Design review of the part shown in the three views and the two pictorial views. Dimensions are in mm from the part's minimum x, y and z. A direction names the side the tool comes from. Give positions to 0.01 mm unless a question says otherwise; leave off trailing zeros. Order: outer loops, then holes, each group sorted by start corner. A loop starts at its lowest first (then second) coordinate and runs counter-clockwise, first axis right, second up.
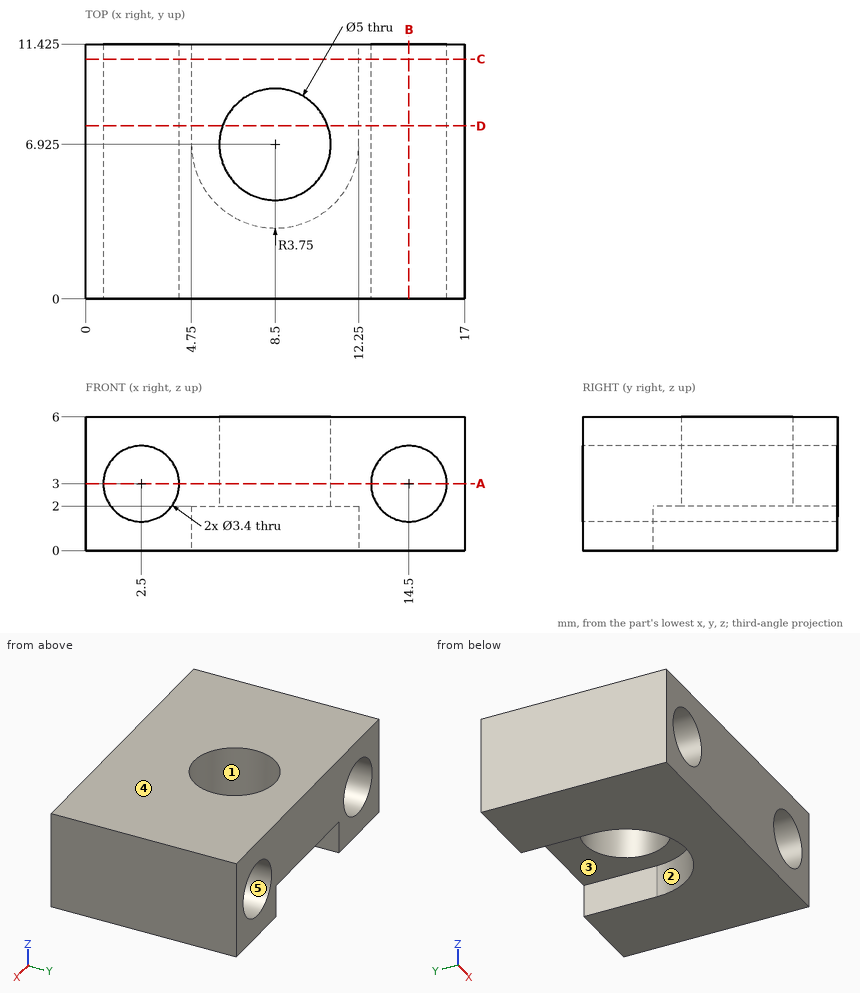
1) Tool access review of the marked faces 1 and 2: name each direction out of +Z, -Z, +X, -X, +Y, -Y from which nothing blocks a thin tool from reaching the whole face with its end or side.
Answer sheet:
face 1: +Z, -Z
face 2: -Z, +Y
2) To check wall thickness, follow line 1 (Z direction, x = 14.5, y = 6.25); line 2 (X direction, y = 5, z = 4.2); line 3 (X direction, y = 5, z = 2.5). State the ranges of each line that lie inside material, in increasing order.
Answer sheet:
line 1: z = 0 to 1.3, 4.7 to 6
line 2: x = 0 to 1.3, 3.7 to 6.9, 10.1 to 13.3, 15.7 to 17
line 3: x = 0 to 0.88, 4.12 to 6.9, 10.1 to 12.88, 16.12 to 17
3) Draft analysis for pull direction Z (two halves, no side actions). For the marked faces 3, 4 and 5, state which applies: +Z half, -Z half, draft (parallel to the pull), parting line (faces both ways), or undercut.
Answer sheet:
face 3: -Z half
face 4: +Z half
face 5: undercut
4) Clearance check with a flat-ended pin moving along its axis: pin 1 (1.5 mm diameter, centred on x = 6, y = 10, fed in from -Z). State where the tip first meets the part, or that it passes through.
Answer sheet:
pin 1: stops at z = 2
5) We need section D-D on y = 7.75. Give the boundary of the cut face in (x, z).
Answer sheet:
outline: (0, 0) - (4.75, 0) - (4.75, 2) - (6.14, 2) - (6.14, 6) - (0, 6) - close; (10.86, 2) - (12.25, 2) - (12.25, 0) - (17, 0) - (17, 6) - (10.86, 6) - close; hole circle Ø3.4 at (2.5, 3); hole circle Ø3.4 at (14.5, 3)
6) We need section A-A on z = 3. Give the boundary of the cut face in (x, y) (3 decimals).
Answer sheet:
outline: (0, 0) - (0.8, 0) - (0.8, 11.425) - (0, 11.425) - close; (4.2, 0) - (12.8, 0) - (12.8, 11.425) - (4.2, 11.425) - close; (16.2, 0) - (17, 0) - (17, 11.425) - (16.2, 11.425) - close; hole circle Ø5 at (8.5, 6.925)
7) We need section C-C on y = 10.75. Give the boundary of the cut face in (x, z), then the cut area to 3 significant figures.
Answer sheet:
outline: (0, 0) - (4.75, 0) - (4.75, 2) - (12.25, 2) - (12.25, 0) - (17, 0) - (17, 6) - (0, 6) - close; hole circle Ø3.4 at (2.5, 3); hole circle Ø3.4 at (14.5, 3)
area: 68.8 mm2
8) We need section B-B on x = 14.5. Give the boundary of the cut face in (y, z) (3 decimals), then the cut area to 3 significant figures.
Answer sheet:
outline: (0, 0) - (11.425, 0) - (11.425, 1.3) - (0, 1.3) - close; (0, 4.7) - (11.425, 4.7) - (11.425, 6) - (0, 6) - close
area: 29.7 mm2
